from build123d import *

# Parameters (mm, degrees)
CROQUIS1_R                 = 0.5
CROQUIS1_R_2               = 1.5
CROQUIS1_W                 = 6
CROQUIS1_H                 = 3
SALIENTE_EXTRUIR1_DEPTH    = 3
S_LIDO_MOVER_COPIAR1_ANGLE = 90


with BuildPart() as part:
    # Croquis1 → Saliente-Extruir1 (new body)
    with BuildSketch(Plane.XY):
        with BuildLine():
            Line((41932.264601563, -390.210765183), (41903.066277894, -389.706454081))
            ThreePointArc((41903.066277894, -389.706454081), (41901.568434997, -389.516485634), (41900.165439728, -388.958609632))
            ThreePointArc((41900.165439728, -388.958609632), (41897.263118587, -388.210765367), (41894.361167478, -388.960044231))
            ThreePointArc((41894.361167478, -388.960044231), (41892.97663061, -389.513886246), (41891.498273009, -389.709186322))
            Line((41891.498273009, -389.709186322), (41817.264601562, -390.210765183))
            ThreePointArc((41817.264601562, -390.210765183), (41813.264601563, -394.210765183), (41817.264601563, -398.210765183))
            Line((41817.264601563, -398.210765183), (41891.457733394, -398.712207088))
            ThreePointArc((41891.457733394, -398.712207088), (41892.957012268, -398.902545922), (41894.361167478, -399.461486136))
            ThreePointArc((41894.361167478, -399.461486136), (41897.263118587, -400.210765), (41900.165439728, -399.462920735))
            ThreePointArc((41900.165439728, -399.462920735), (41901.518409746, -398.918171578), (41902.962844991, -398.715967883))
            Line((41902.962844991, -398.715967883), (41932.264601563, -398.210765183))
            ThreePointArc((41932.264601563, -398.210765183), (41936.264601563, -394.210765183), (41932.264601563, -390.210765183))
        make_face()
        with Locations((41817.264601563, -394.210765183)):
            Circle(CROQUIS1_R, mode=Mode.SUBTRACT)
        with Locations((41932.264601563, -394.210765183)):
            Circle(CROQUIS1_R_2, mode=Mode.SUBTRACT)
        with Locations((41897.264601563, -394.210765183)):
            Circle(CROQUIS1_R_2, mode=Mode.SUBTRACT)
        with Locations((41859.764601563, -392.210765183)):
            Rectangle(CROQUIS1_W, CROQUIS1_H, mode=Mode.SUBTRACT)
    extrude(amount=SALIENTE_EXTRUIR1_DEPTH)


with BuildPart() as part_1:
    # Sólido-Mover/Copiar1: moved
    add(part.part.rotate(Axis((0, -394.210765183, 1.5), (-1, 0, 0)), S_LIDO_MOVER_COPIAR1_ANGLE))


solid = part_1.part
Part model, mm, in its own coordinate system. A direction names the side the tool comes from. Coordinates: 2 decimals unless noted, no trailing zeros. Write each loop counter-clockwise with the first axis right and the second up, starting at its lowest first coordinate (ties: lowest second). Pieces come first, ordered by that corner, then holes. Notation, with made-up numbers: (-10, 43.25) - (32, 43.25) arc R26 ccw to (32, 70.25) - close; hole circle Ø4 at (-5, -6). An arc over 180 degrees is marked (long way). Put each result on its own line as item: value.
1. Flat gauge pins, fed straight in: pin 1 Ø0.9 at (x, y) = (41860.5, -395) entering from -Z; pin 2 Ø0.9 at (x, y) = (41860, -394) entering from +Z; pin 3 Ø1 at (x, y) = (41826, -394.5) entering from +Z. Where does each tip first touch, or does it go through?
Final values:
pin 1: stops at z = -2.8
pin 2: stops at z = 5.79
pin 3: stops at z = 5.56
2. Probe line 1 along X through (y, z) = (-394.65, 1.5); line 2 along Z through (x, y) = (41820, -393.6); line 3 along X through (y, z) = (-394.3, -1.5). List the from-to ranges inside material, lowest first. Write a range as [from, to].
Final values:
line 1: x = [41813.26, 41816.76], [41817.76, 41895.76], [41898.76, 41930.76], [41933.76, 41936.26]
line 2: z = [-2.52, 5.52]
line 3: x = [41814.62, 41856.76], [41862.76, 41934.91]
3. Band-saw the part on C-C (x = 41888). Write the cut outline in (y, z), then the cut area to 3 significant figures.
Final values:
outline: (-395.71, -2.98) - (-392.71, -2.98) - (-392.71, 5.98) - (-395.71, 5.98) - close
area: 26.9 mm²
4. Band-saw the part on A-A (y = -394.7). Write the cut outline in (x, z), then the cut area to 3 significant figures.
Final values:
outline: (41817.26, -2.5) - (41891.5, -3) arc R6 cw to (41894.36, -3.75) arc R6 ccw to (41900.17, -3.75) arc R6 cw to (41903.07, -3) - (41932.26, -2.5) arc R4 ccw to (41932.26, 5.5) - (41902.96, 6.01) arc R6 cw to (41900.17, 6.75) arc R6 ccw to (41894.36, 6.75) arc R6 cw to (41891.46, 6) - (41817.26, 5.5) arc R4 ccw to start; hole circle Ø1 at (41817.26, 1.5); hole (41856.76, -2) - (41862.76, -2) - (41862.76, 1) - (41856.76, 1) - close; hole circle Ø3 at (41897.26, 1.5); hole circle Ø3 at (41932.26, 1.5)
area: 1,020 mm²
5. Two-plate mould, pull along X, no slides. Class faces 3 (the cylindrical face through (41813.266, -394.232, 1.412)), 4 (the flat face through (41860, -394, -2)), 5 (the flat face through (41874, -395.711, 1)): +X half, -X half, draft (parallel to the pull), parting line (faces both ways), or undercut.
Final values:
face 3: -X half
face 4: undercut
face 5: draft
6. 3-axis set-ups, long thin cutter, end or side, ignore diameter. For faces 1 (the flat face through (41860, -394, 1)), 2 (the cylindrical face through (41936.264, -394.232, 1.588)): which of +Z, -Z, +X, -X, +Y, -Y reach the whole face in a straight line?
Final values:
face 1: +Y, -Y
face 2: +X, +Y, -Y
7. Band-saw the part on B-B (x = 41875). Write the cut outline in (y, z), then the cut area to 3 significant figures.
Final values:
outline: (-395.71, -2.89) - (-392.71, -2.89) - (-392.71, 5.89) - (-395.71, 5.89) - close
area: 26.3 mm²
